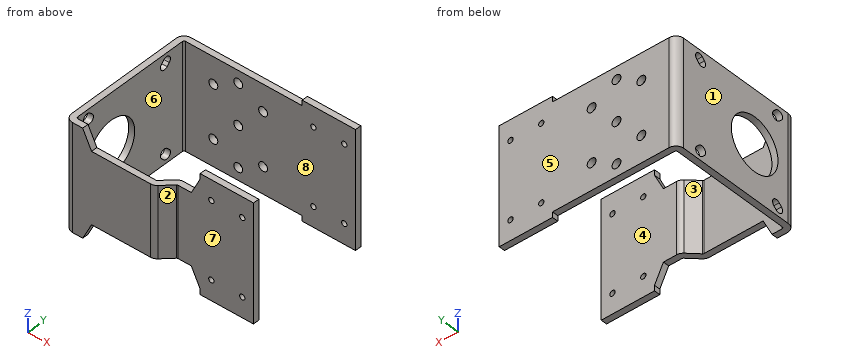
```python
from build123d import *

# Parameters (mm, degrees)
BASE_FLANGE1_DEPTH             = 60
SKETCH6_R                      = 15
CUT_EXTRUDE1_DEPTH             = 3.4
CUT_EXTRUDE2_START             = -65
CUT_EXTRUDE2_OUTLINE_W         = 10
CUT_EXTRUDE2_OUTLINE_H         = 10.4
CUT_EXTRUDE2_DEPTH             = 50
SKETCH10_W                     = 3
SKETCH10_H                     = 3.4
BOSS_EXTRUDE1_DEPTH            = 30
MIRROR2_COPY_1_SKETCH_W        = 3
MIRROR2_COPY_1_SKETCH_H        = 3.4
MIRROR2_COPY_1_DEPTH           = 30
SKETCH13_R                     = 1.5
CUT_EXTRUDE3_DEPTH             = 141.516902898
CUT_EXTRUDE6_REACH             = 142.517
SKETCH14_R                     = 2.5
CUT_EXTRUDE7_DEPTH             = 5
CUT_EXTRUDE7_DIRECTION_2_REACH = 138.858


# Read off the part's stored shape, not the designer's step: Cut-Extrude2
# Sheet-metal steps are written as plain solids
with BuildPart() as part:
    # Sketch1 → Base-Flange1 (new body)
    with BuildSketch(Plane.XY):
        with BuildLine():
            Line((100, 0), (4.4, 0))
            ThreePointArc((4.4, 0), (1.288730163, -1.288730163), (0, -4.4))
            Line((0, -4.4), (0, -71.6))
            ThreePointArc((0, -71.6), (1.288730163, -74.711269837), (4.4, -76))
            Line((4.4, -76), (48.203183584, -76))
            ThreePointArc((48.203183584, -76), (49.866643015, -75.673438685), (51.283183584, -74.742228509))
            Line((51.283183584, -74.742228509), (56.849795796, -69.285857157))
            ThreePointArc((56.849795796, -69.285857157), (57.171736834, -69.074218481), (57.549795796, -69))
            Line((57.549795796, -69), (100, -69))
            Line((100, -69), (100, -65.6))
            Line((100, -65.6), (57.549795796, -65.6))
            ThreePointArc((57.549795796, -65.6), (55.886336364, -65.926561315), (54.469795796, -66.857771491))
            Line((54.469795796, -66.857771491), (48.903183584, -72.314142843))
            ThreePointArc((48.903183584, -72.314142843), (48.581242545, -72.525781519), (48.203183584, -72.6))
            Line((48.203183584, -72.6), (4.4, -72.6))
            ThreePointArc((4.4, -72.6), (3.692893219, -72.307106781), (3.4, -71.6))
            Line((3.4, -71.6), (3.4, -4.4))
            ThreePointArc((3.4, -4.4), (3.692893219, -3.692893219), (4.4, -3.4))
            Line((4.4, -3.4), (100, -3.4))
            Line((100, -3.4), (100, 0))
        make_face()
    extrude(amount=BASE_FLANGE1_DEPTH)

    # Sketch6 → Cut-Extrude1 (cut)
    with BuildSketch(Plane.ZY):
        with Locations(Location((30, -50, 0), (0, 0, 270))):
            Circle(SKETCH6_R)
        with BuildLine():
            Line((57.224873734, -63.689339828), (55.810660172, -62.275126266))
            ThreePointArc((55.810660172, -62.275126266), (52.275126266, -62.275126266), (52.275126266, -65.810660172))
            Line((52.275126266, -65.810660172), (53.689339828, -67.224873734))
            ThreePointArc((53.689339828, -67.224873734), (57.224873734, -67.224873734), (57.224873734, -63.689339828))
        make_face()
        with BuildLine():
            Line((2.775126266, -16.310660172), (4.189339828, -17.724873734))
            ThreePointArc((4.189339828, -17.724873734), (7.724873734, -17.724873734), (7.724873734, -14.189339828))
            Line((7.724873734, -14.189339828), (6.310660172, -12.775126266))
            ThreePointArc((6.310660172, -12.775126266), (2.775126266, -12.775126266), (2.775126266, -16.310660172))
        make_face()
        with BuildLine():
            Line((53.689339828, -12.775126266), (52.275126266, -14.189339828))
            ThreePointArc((52.275126266, -14.189339828), (52.275126266, -17.724873734), (55.810660172, -17.724873734))
            Line((55.810660172, -17.724873734), (57.224873734, -16.310660172))
            ThreePointArc((57.224873734, -16.310660172), (57.224873734, -12.775126266), (53.689339828, -12.775126266))
        make_face()
        with BuildLine():
            Line((6.310660172, -67.224873734), (7.724873734, -65.810660172))
            ThreePointArc((7.724873734, -65.810660172), (7.724873734, -62.275126266), (4.189339828, -62.275126266))
            Line((4.189339828, -62.275126266), (2.775126266, -63.689339828))
            ThreePointArc((2.775126266, -63.689339828), (2.775126266, -67.224873734), (6.310660172, -67.224873734))
        make_face()
    extrude(amount=-CUT_EXTRUDE1_DEPTH, mode=Mode.SUBTRACT)

    # Cut-Extrude2 outline → Cut-Extrude2 (cut)
    with BuildSketch(Plane.ZY.offset(CUT_EXTRUDE2_START)):
        with Locations((55, -70.8)):
            Rectangle(CUT_EXTRUDE2_OUTLINE_W, CUT_EXTRUDE2_OUTLINE_H)
        with Locations((5, -70.8)):
            Rectangle(CUT_EXTRUDE2_OUTLINE_W, CUT_EXTRUDE2_OUTLINE_H)
    extrude(amount=CUT_EXTRUDE2_DEPTH, mode=Mode.SUBTRACT)

    # Sketch10 → Boss-Extrude1 (add)
    with BuildSketch(Plane(origin=(100, 0, 0), x_dir=(0, 0, -1), z_dir=(1, 0, 0))):
        with Locations((1.5, -1.7)):
            Rectangle(SKETCH10_W, SKETCH10_H)
    boss_extrude1 = extrude(amount=-BOSS_EXTRUDE1_DEPTH)

    # Mirror1: Boss-Extrude1 across plane
    add(boss_extrude1.mirror(Plane(origin=(0, 0, 30), x_dir=(1, 0, 0), z_dir=(0, 0, -1))))

    # Mirror2: Boss-Extrude1 across plane
    add(boss_extrude1.mirror(Plane(origin=(0, -34.5, 0), x_dir=(0, 0, 1), z_dir=(0, -1, 0))))

    # Mirror2 copy 1 sketch → Mirror2 copy 1 (add)
    with BuildSketch(Plane(origin=(100, -69, 60), x_dir=(0, 0, 1), z_dir=(1, 0, 0))):
        with Locations((1.5, -1.7)):
            Rectangle(MIRROR2_COPY_1_SKETCH_W, MIRROR2_COPY_1_SKETCH_H)
    extrude(amount=-MIRROR2_COPY_1_DEPTH)

    # Sketch13 → Cut-Extrude3 (cut, through all)
    with BuildSketch(Plane(origin=(0, 0, 0), x_dir=(1, 0, 0), z_dir=(0, 1, 0))):
        with Locations(Location((76.306667563, -8.329371406, 0), (0, 0, 270))):
            Circle(SKETCH13_R)
        with Locations(Location((93.693332437, -8.329371406, 0), (0, 0, 270))):
            Circle(SKETCH13_R)
    cut_extrude3 = extrude(amount=-CUT_EXTRUDE3_DEPTH, mode=Mode.SUBTRACT)

    # Mirror3: Cut-Extrude3 across plane
    add(cut_extrude3.mirror(Plane(origin=(0, 0, 30), x_dir=(1, 0, 0), z_dir=(0, 0, -1))), mode=Mode.SUBTRACT)

    # Sketch14 → Cut-Extrude6 (cut, up to next)
    with BuildSketch(Plane(origin=(0, 0, 0), x_dir=(1, 0, 0), z_dir=(0, 1, 0)), mode=Mode.PRIVATE) as cut_extrude6_sk1:
        with Locations(Location((20, -15, 0), (0, 0, 270))):
            Circle(SKETCH14_R)
    cut_extrude6_tool1 = extrude(cut_extrude6_sk1.sketch, amount=-CUT_EXTRUDE6_REACH, mode=Mode.PRIVATE) & part.part
    # Sketch14 → Cut-Extrude6 (cut, up to next)
    with BuildSketch(Plane(origin=(0, 0, 0), x_dir=(1, 0, 0), z_dir=(0, 1, 0)), mode=Mode.PRIVATE) as cut_extrude6_sk2:
        with Locations(Location((48, -15, 0), (0, 0, 270))):
            Circle(SKETCH14_R)
    cut_extrude6_tool2 = extrude(cut_extrude6_sk2.sketch, amount=-CUT_EXTRUDE6_REACH, mode=Mode.PRIVATE) & part.part
    # Sketch14 → Cut-Extrude6 (cut, up to next)
    with BuildSketch(Plane(origin=(0, 0, 0), x_dir=(1, 0, 0), z_dir=(0, 1, 0)), mode=Mode.PRIVATE) as cut_extrude6_sk3:
        with Locations(Location((48, -45, 0), (0, 0, 270))):
            Circle(SKETCH14_R)
    cut_extrude6_tool3 = extrude(cut_extrude6_sk3.sketch, amount=-CUT_EXTRUDE6_REACH, mode=Mode.PRIVATE) & part.part
    # Sketch14 → Cut-Extrude6 (cut, up to next)
    with BuildSketch(Plane(origin=(0, 0, 0), x_dir=(1, 0, 0), z_dir=(0, 1, 0)), mode=Mode.PRIVATE) as cut_extrude6_sk4:
        with Locations(Location((20, -45, 0), (0, 0, 270))):
            Circle(SKETCH14_R)
    cut_extrude6_tool4 = extrude(cut_extrude6_sk4.sketch, amount=-CUT_EXTRUDE6_REACH, mode=Mode.PRIVATE) & part.part
    # Sketch14 → Cut-Extrude6 (cut, up to next)
    with BuildSketch(Plane(origin=(0, 0, 0), x_dir=(1, 0, 0), z_dir=(0, 1, 0)), mode=Mode.PRIVATE) as cut_extrude6_sk5:
        with Locations(Location((34, -30, 0), (0, 0, 270))):
            Circle(SKETCH14_R)
    cut_extrude6_tool5 = extrude(cut_extrude6_sk5.sketch, amount=-CUT_EXTRUDE6_REACH, mode=Mode.PRIVATE) & part.part
    # Sketch14 → Cut-Extrude6 (cut, up to next)
    with BuildSketch(Plane(origin=(0, 0, 0), x_dir=(1, 0, 0), z_dir=(0, 1, 0)), mode=Mode.PRIVATE) as cut_extrude6_sk6:
        with Locations(Location((34, -7, 0), (0, 0, 270))):
            Circle(SKETCH14_R)
    cut_extrude6_tool6 = extrude(cut_extrude6_sk6.sketch, amount=-CUT_EXTRUDE6_REACH, mode=Mode.PRIVATE) & part.part
    # Sketch14 → Cut-Extrude6 (cut, up to next)
    with BuildSketch(Plane(origin=(0, 0, 0), x_dir=(1, 0, 0), z_dir=(0, 1, 0)), mode=Mode.PRIVATE) as cut_extrude6_sk7:
        with Locations(Location((34, -53, 0), (0, 0, 270))):
            Circle(SKETCH14_R)
    cut_extrude6_tool7 = extrude(cut_extrude6_sk7.sketch, amount=-CUT_EXTRUDE6_REACH, mode=Mode.PRIVATE) & part.part
    add(cut_extrude6_tool1.solids().sort_by_distance((20, 0, 15))[0], mode=Mode.SUBTRACT)
    add(cut_extrude6_tool2.solids().sort_by_distance((48, 0, 15))[0], mode=Mode.SUBTRACT)
    add(cut_extrude6_tool3.solids().sort_by_distance((48, 0, 45))[0], mode=Mode.SUBTRACT)
    add(cut_extrude6_tool4.solids().sort_by_distance((20, 0, 45))[0], mode=Mode.SUBTRACT)
    add(cut_extrude6_tool5.solids().sort_by_distance((34, 0, 30))[0], mode=Mode.SUBTRACT)
    add(cut_extrude6_tool6.solids().sort_by_distance((34, 0, 7))[0], mode=Mode.SUBTRACT)
    add(cut_extrude6_tool7.solids().sort_by_distance((34, 0, 53))[0], mode=Mode.SUBTRACT)

    # Sketch15 → Cut-Extrude7 (cut)
    with BuildSketch(Plane.XZ.offset(69)):
        Polygon((65, 50), (70, 60), (65, 60), align=None)
        Polygon((15, 50), (15, 60), (10, 60), align=None)
    cut_extrude7 = extrude(amount=-CUT_EXTRUDE7_DEPTH, mode=Mode.SUBTRACT)

    # Cut-Extrude7 direction 2: up to this face of the body (flat: up to its plane)
    cut_extrude7_direction_2_end = Plane(part.part.faces().sort_by_distance((24.509682794, -76, 30))[0])
    # Sketch15 → Cut-Extrude7 direction 2 (cut, up to the picked face)
    with BuildSketch(Plane.XZ.offset(69), mode=Mode.PRIVATE) as cut_extrude7_direction_2_sk1:
        Polygon((65, 50), (70, 60), (65, 60), align=None)
    cut_extrude7_direction_2_tool1 = split(extrude(cut_extrude7_direction_2_sk1.sketch, amount=CUT_EXTRUDE7_DIRECTION_2_REACH, mode=Mode.PRIVATE), bisect_by=cut_extrude7_direction_2_end, keep=Keep.BOTH, mode=Mode.PRIVATE)
    # Sketch15 → Cut-Extrude7 direction 2 (cut, up to the picked face)
    with BuildSketch(Plane.XZ.offset(69), mode=Mode.PRIVATE) as cut_extrude7_direction_2_sk2:
        Polygon((15, 50), (15, 60), (10, 60), align=None)
    cut_extrude7_direction_2_tool2 = split(extrude(cut_extrude7_direction_2_sk2.sketch, amount=CUT_EXTRUDE7_DIRECTION_2_REACH, mode=Mode.PRIVATE), bisect_by=cut_extrude7_direction_2_end, keep=Keep.BOTH, mode=Mode.PRIVATE)
    cut_extrude7_direction_2_1 = cut_extrude7_direction_2_tool1.solids().sort_by(Axis((66.666667, -69, 56.666667), (0, -1, 0)))[0]
    add(cut_extrude7_direction_2_1, mode=Mode.SUBTRACT)
    cut_extrude7_direction_2_2 = cut_extrude7_direction_2_tool2.solids().sort_by(Axis((13.333333, -69, 56.666667), (0, -1, 0)))[0]
    add(cut_extrude7_direction_2_2, mode=Mode.SUBTRACT)
    cut_extrude7_direction_2 = cut_extrude7_direction_2_1 + cut_extrude7_direction_2_2  # Cut-Extrude7 direction 2 as one shape, for the pattern or mirror that repeats it

    # Mirror4: Cut-Extrude7, Cut-Extrude7 direction 2 across plane
    add(cut_extrude7.mirror(Plane(origin=(0, 0, 30), x_dir=(1, 0, 0), z_dir=(0, 0, -1))), mode=Mode.SUBTRACT)
    add(cut_extrude7_direction_2.mirror(Plane(origin=(0, 0, 30), x_dir=(1, 0, 0), z_dir=(0, 0, -1))), mode=Mode.SUBTRACT)


solid = part.part
```
Source: CAD feature listing. Evaluate the final solid. Frame: model axes, mm. Face numbers are marked on the shaded views. A direction names the side the tool comes from. Give positions to 0.01 mm unless a question says otherwise; leave off trailing zeros. Loops run counter-clockwise (first coordinate to the right, second up) from the corner with the lowest first, then second, coordinate; pieces in that order, holes last. Notation, with made-up numbers: (48.25, 1) - (73.25, 1) arc R21 ccw to (73.25, 29) - close; hole circle Ø7 at (16, 19.5). An arc over 180 degrees is marked (long way). Use CSV: the item, a comma, the result in double quotes. Start each with the question number.
1. Section B-B (y = -50). Output: boundary loops of the cut face in (x, z), then the cut area to 3 significant figures.
2. Ray query, L1, parallel to Y at x = 7, z = 48.5; L2, parallel to Y at x = 72, z = 38.5; L3, parallel to X at y = -0.8, z = 53. Return the intervals inside material, ascending.
3. Reachability of the marked faces 5, 6, 7 and 8 from +Z, -Z, +X, -X, +Y, -Y: full face, straight path, thin tool, end or side. Return the list, or none.
4. Section D-D (y = -27). Output: boundary loops of the cut face in (x, z), then the cut area to 3 significant figures.
5. Draft query along X for the marked faces 1, 2, 3 and 4. Return one class per face: +X half, -X half, draft (parallel to the pull), parting line (faces both ways), or undercut.
6. Section A-A (x = 12). Output: boundary loops of the cut face in (y, z).
7. Pin query (flat end, axial travel): pin 1 (2 mm diameter, centred on x = 82, z = 12, fed in from -Y); pin 2 (11.5 mm diameter, centred on x = 52, y = -69.5, fed in from +Z); pin 3 (1 mm diameter, centred on y = -45, z = 15.5, fed in from +X). Return the tip coordinate at first contact, or that it passes through.
8. Section C-C (x = 34). Output: boundary loops of the cut face in (y, z), then the cut area to 3 significant figures.
Response:
1,outline,"(0, 0) - (3.4, 0) - (3.4, 15) - (0, 15) - close; (0, 45) - (3.4, 45) - (3.4, 60) - (0, 60) - close"
1,area,"102 mm²"
2,L1,"-76 to -72.6, -3.4 to 0"
2,L2,"-69 to -65.6, -3.4 to 0"
2,L3,"1.87 to 31.5, 36.5 to 75.61, 77 to 93, 94.39 to 100"
3,face 5,"+Z, -Z, +X, -X, +Y"
3,face 6,"+Z, -Z"
3,face 7,"+Z, -Z, +X, -Y"
3,face 8,"+Z, -Z, +X"
4,outline,"(0, 0) - (3.4, 0) - (3.4, 60) - (0, 60) - close"
4,area,"204 mm²"
5,face 1,"-X half"
5,face 2,"+X half"
5,face 3,"undercut"
5,face 4,"draft"
6,outline,"(-76, 4) - (-72.6, 4) - (-72.6, 56) - (-76, 56) - close; (-3.4, 0) - (0, 0) - (0, 60) - (-3.4, 60) - close"
7,pin 1,"y = -69"
7,pin 2,"z = 50"
7,pin 3,"x = 3.4"
8,outline,"(-76, 10) - (-72.6, 10) - (-72.6, 50) - (-76, 50) - close; (-3.4, 0) - (0, 0) - (0, 4.5) - (-3.4, 4.5) - close; (-3.4, 9.5) - (0, 9.5) - (0, 27.5) - (-3.4, 27.5) - close; (-3.4, 32.5) - (0, 32.5) - (0, 50.5) - (-3.4, 50.5) - close; (-3.4, 55.5) - (0, 55.5) - (0, 60) - (-3.4, 60) - close"
8,area,"289 mm²"
